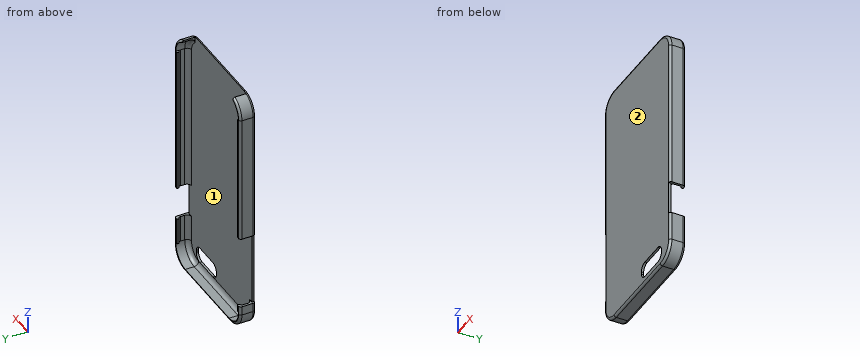
from build123d import *

# Parameters (mm, degrees)
SKETCH1_W           = 70.104
SKETCH1_H           = 140.716
BOSS_EXTRUDE1_DEPTH = 1.27
SKETCH2_W           = 67.564
SKETCH2_H           = 138.176
BOSS_EXTRUDE2_DEPTH = 7.62
SKETCH3_W           = 41.91
SKETCH3_H           = 7.62
CUT_EXTRUDE1_DEPTH  = 1.27
SKETCH5_W           = 19.05
SKETCH5_H           = 7.62
CUT_EXTRUDE2_DEPTH  = 1.27
SKETCH6_W           = 54.864
SKETCH6_H           = 7.62
CUT_EXTRUDE3_DEPTH  = 1.27
SKETCH7_W           = 21.59
SKETCH7_H           = 8.89
CUT_EXTRUDE4_DEPTH  = 1.27
FILLET1_R           = 10.16
FILLET2_R           = 10.16
SKETCH8_W           = 3.81
SKETCH8_H           = 1.27
BOSS_EXTRUDE3_DEPTH = 1.27
SKETCH14_W          = 15.24
SKETCH14_H          = 1.27
BOSS_EXTRUDE7_DEPTH = 1.27
SKETCH19_W          = 84.307427921
SKETCH19_H          = 1.27
BOSS_EXTRUDE8_DEPTH = 1.27
SKETCH20_W          = 72.877427921
SKETCH20_H          = 1.27
BOSS_EXTRUDE9_DEPTH = 1.27
FILLET9_R           = 3.81
FILLET12_R          = 1.27
FILLET15_R          = 1.27
FILLET16_R          = 2.54
SKETCH28_W          = 1.27
SKETCH28_H          = 19.05
SKETCH28_H_2        = 41.91
CUT_EXTRUDE10_DEPTH = 1.27
FILLET18_R          = 1.27


# Some blends are built 0.0001 mm under size
with BuildPart() as part:
    # Sketch1 → Boss-Extrude1 (new body)
    with BuildSketch(Plane(origin=(0, 0, 0), x_dir=(1, 0, 0), z_dir=(0, 1, 0))):
        Rectangle(SKETCH1_W, SKETCH1_H)
    extrude(amount=BOSS_EXTRUDE1_DEPTH)

    # Sketch2 → Boss-Extrude2 (add)
    with BuildSketch(Plane(origin=(0, 1.27, 0), x_dir=(1, 0, 0), z_dir=(0, 1, 0))):
        Polygon((-35.052, -70.358), (0, -70.358), (35.052, -70.358), (35.052, 70.358), (-35.052, 70.358), align=None)
        Rectangle(SKETCH2_W, SKETCH2_H, mode=Mode.SUBTRACT)
    extrude(amount=BOSS_EXTRUDE2_DEPTH)

    # Sketch3 → Cut-Extrude1 (cut)
    with BuildSketch(Plane.ZY.offset(35.052)):
        with Locations((-34.163, 5.08)):
            Rectangle(SKETCH3_W, SKETCH3_H)
    extrude(amount=-CUT_EXTRUDE1_DEPTH, mode=Mode.SUBTRACT)

    # Sketch5 → Cut-Extrude2 (cut)
    with BuildSketch(Plane(origin=(35.052, 0, 0), x_dir=(0, 0, -1), z_dir=(1, 0, 0))):
        with Locations((34.163, 5.08)):
            Rectangle(SKETCH5_W, SKETCH5_H)
    extrude(amount=-CUT_EXTRUDE2_DEPTH, mode=Mode.SUBTRACT)

    # Sketch6 → Cut-Extrude3 (cut)
    with BuildSketch(Plane.XY.offset(70.358)):
        with Locations((0, 5.08)):
            Rectangle(SKETCH6_W, SKETCH6_H)
    extrude(amount=-CUT_EXTRUDE3_DEPTH, mode=Mode.SUBTRACT)

    # Sketch7 → Cut-Extrude4 (cut)
    with BuildSketch(Plane.XZ):
        with Locations((15.367, -62.103)):
            Rectangle(SKETCH7_W, SKETCH7_H)
    extrude(amount=-CUT_EXTRUDE4_DEPTH, mode=Mode.SUBTRACT)

    # Fillet1
    # the kernel refuses this fillet: 10.16 mm, written as the material it adds along each edge
    with BuildSketch(Plane(origin=(33.782, 1.27, -69.088), x_dir=(0, 0, 1), z_dir=(0, 1, 0)), Plane(origin=(-33.782, 1.27, -69.088), x_dir=(1, 0, 0), z_dir=(0, 1, 0))) as fillet1_piece_1:
        with BuildLine():
            CenterArc((FILLET1_R, -FILLET1_R), FILLET1_R, 90, 90)
            Line((0, -FILLET1_R), (-FILLET1_R * 0.02, -FILLET1_R))
            Line((-FILLET1_R * 0.02, -FILLET1_R), (-FILLET1_R * 0.02, FILLET1_R * 0.02))
            Line((-FILLET1_R * 0.02, FILLET1_R * 0.02), (FILLET1_R, FILLET1_R * 0.02))
            Line((FILLET1_R, FILLET1_R * 0.02), (FILLET1_R, 0))
        make_face()
    extrude(amount=7.62)
    with BuildSketch(Plane(origin=(-33.782, 1.27, 69.088), x_dir=(0, 0, -1), z_dir=(0, 1, 0))) as fillet1_piece_2:
        with BuildLine():
            CenterArc((9.418572079, -10.16), FILLET1_R, 90, 67.975687163)
            Line((0, -6.35), (-0.188371442, -6.2738))
            ThreePointArc((-0.188371442, -6.2738), (-0.2032, -3.175), (-0.2032, 0))
            Line((-0.2032, 0), (0, 0.2032))
            Line((0, 0.2032), (9.418572079, 0.2032))
            Line((9.418572079, 0.2032), (9.418572079, 0))
        make_face()
    extrude(amount=7.62)
    with BuildSketch(Plane(origin=(33.782, 1.27, 69.088), x_dir=(-1, 0, 0), z_dir=(0, 1, 0))) as fillet1_piece_3:
        with BuildLine():
            CenterArc((10.16, -9.418572079), FILLET1_R, 112.024312837, 67.975687163)
            Line((0, -9.418572079), (-0.2032, -9.418572079))
            Line((-0.2032, -9.418572079), (-0.2032, 0))
            Line((-0.2032, 0), (0, 0.2032))
            ThreePointArc((0, 0.2032), (3.175, 0.2032), (6.2738, 0.188371442))
            Line((6.2738, 0.188371442), (6.35, 0))
        make_face()
    extrude(amount=7.62)

    # Fillet2
    fillet2_edges = [part.edges().sort_by_distance(p)[0] for p in [
        (-35.052, 4.445, -70.358),
        (35.052, 4.445, -70.358),
        (35.052, 4.445, 70.358),
        (-35.052, 4.445, 70.358),
    ]]
    fillet(fillet2_edges, radius=FILLET2_R)

    # Sketch8 → Boss-Extrude3 (add)
    with BuildSketch(Plane(origin=(-33.782, 0, 0), x_dir=(0, 0, -1), z_dir=(1, 0, 0))):
        with Locations((57.023, 8.255)):
            Rectangle(SKETCH8_W, SKETCH8_H)
    extrude(amount=BOSS_EXTRUDE3_DEPTH)

    # Sketch14 → Boss-Extrude7 (add)
    with BuildSketch(Plane.ZY.offset(-33.782)):
        with Locations((-51.308, 8.255)):
            Rectangle(SKETCH14_W, SKETCH14_H)
    extrude(amount=BOSS_EXTRUDE7_DEPTH)

    # Sketch19 → Boss-Extrude8 (add)
    with BuildSketch(Plane.ZY.offset(-33.782)):
        with Locations((17.515713961, 8.255)):
            Rectangle(SKETCH19_W, SKETCH19_H)
    extrude(amount=BOSS_EXTRUDE8_DEPTH)

    # Sketch20 → Boss-Extrude9 (add)
    with BuildSketch(Plane(origin=(-33.782, 0, 0), x_dir=(0, 0, -1), z_dir=(1, 0, 0))):
        with Locations((-23.230713961, 8.255)):
            Rectangle(SKETCH20_W, SKETCH20_H)
    extrude(amount=BOSS_EXTRUDE9_DEPTH)

    # Fillet9
    fillet9_edges = [part.edges().sort_by_distance(p)[0] for p in [
        (26.162, 0.635, -57.658),
        (26.162, 0.635, -66.548),
        (4.572, 0.635, -66.548),
        (4.572, 0.635, -57.658),
    ]]
    fillet(fillet9_edges, radius=FILLET9_R)

    # Fillet12
    fillet12_edges = [part.edges().sort_by_distance(p)[0] for p in [
        (32.076204897, 0, 67.382204897),
        (0, 0, 70.358),
        (-32.076204897, 0, 67.382204897),
        (-35.052, 0, 0),
        (-32.076204897, 0, -67.382204897),
        (0, 0, -70.358),
        (32.076204897, 0, -67.382204897),
        (35.052, 0, 0),
    ]]
    fillet(fillet12_edges, radius=FILLET12_R - 0.0001)  # a hair under: the kernel refuses the full size

    # Fillet15
    fillet15_edges = [part.edges().sort_by_distance(p)[0] for p in [
        (-35.052, 8.89, -57.658),
        (0, 8.89, -70.358),
        (-32.076204897, 8.89, -67.382204897),
        (35.052, 8.89, 17.78),
        (-35.052, 8.89, 23.495),
        (32.076204897, 8.89, -67.382204897),
        (32.924185257, 8.89, 66.419703947),
        (-32.924185257, 8.89, 66.419703947),
        (35.052, 8.89, -51.943),
    ]]
    fillet(fillet15_edges, radius=FILLET15_R - 0.0001)  # a hair under: the kernel refuses the full size

    # Fillet16
    fillet16_edges = [part.edges().sort_by_distance(p)[0] for p in [
        (0, 1.27, -69.088),
        (-33.782, 1.27, -57.023),
        (33.782, 1.27, 17.515713961),
        (-30.806204897, 1.27, -66.112204897),
        (30.806204897, 1.27, -66.112204897),
        (32.046226968, 1.27, 65.349040584),
        (-32.046226968, 1.27, 65.349040584),
        (-33.782, 1.27, 23.230713961),
        (33.782, 1.27, -51.308),
    ]]
    fillet(fillet16_edges, radius=FILLET16_R - 0.0001)  # a hair under: the kernel refuses the full size

    # Sketch28 → Cut-Extrude10 (cut)
    with BuildSketch(Plane(origin=(0, 1.27, 0), x_dir=(1, 0, 0), z_dir=(0, 1, 0))):
        with Locations((34.417, 34.163)):
            Rectangle(SKETCH28_W, SKETCH28_H)
        with Locations((-34.417, 34.163)):
            Rectangle(SKETCH28_W, SKETCH28_H_2)
    extrude(amount=-CUT_EXTRUDE10_DEPTH, mode=Mode.SUBTRACT)

    # Fillet18
    fillet18_edges = [part.edges().sort_by_distance(p)[0] for p in [
        (33.782, 7.62, -51.308),
        (-33.782, 7.62, -57.023),
        (33.782, 7.62, 17.515713961),
        (-33.782, 7.62, 23.230713961),
    ]]
    fillet(fillet18_edges, radius=FILLET18_R - 0.0001)  # a hair under: the kernel refuses the full size


solid = part.part
Could you check a few things on this model? Use its own coordinates, in mm. Face numbers are marked on the shaded views. Give positions to 0.01 mm unless a question says otherwise; leave off trailing zeros.
Item 1: I'm going to push flat-ended pins straight in: pin 1 (1.1 mm diameter, centred on x = -32.5, y = 3, fed in from +Z); pin 2 (6 mm diameter, centred on x = -27, z = -30.5, fed in from -Y); pin 3 (1 mm diameter, centred on y = 8.5, z = 22.5, fed in from +X); pin 4 (0.6 mm diameter, centred on y = 8.5, z = 9.5, fed in from -X). Where does each tip first touch, or does it pass through?
Item 2: I need wall thicknesses on line 1 (X direction, y = 5.5, z = 35); line 2 (Y direction, x = 30.5, z = 34); line 3 (X direction, y = 2.75, z = 65). Which ranges of each line are inside material? Lowest first, please.
Item 3: If we mould it in two halves opening along X, with no side actions, what happens to the marked faces 1 and 2? For each: pulls with the +X half, pulls with the -X half, needs draft (parallel to the pull), parting line crosses it, or undercut.
Values:
1. pin 1: stops at z = 67.51
1. pin 2: stops at y = 0
1. pin 3: stops at x = 34.99
1. pin 4: stops at x = -34.91
2. line 1: x = -35.05 to -33.78, 33.78 to 35.05
2. line 2: y = 0 to 1.27
2. line 3: x = -33.85 to -32, 32 to 33.85
3. face 1: undercut
3. face 2: needs draft
